```python
from build123d import *

# Parameters (mm, degrees)
SKETCH_1_R              = 5
EXTRUDE_1_DEPTH         = 10
SKETCH_2_R              = 4.501699131
SKETCH_2_R_2            = 2
CUT_EXTRUDE_1_DEPTH     = 0.5
HOLE_WIZARD_M2_21_D     = 2.3
HOLE_WIZARD_M2_21_DEPTH = 2
HOLE_WIZARD_M2_21_TIP   = 0.690989712


with BuildPart() as part:
    # Эскиз1 → Бобышка-Вытянуть1 (new body)
    with BuildSketch(Plane(origin=(0, 0, 0), x_dir=(1, 0, 0), z_dir=(0, 1, 0))):
        Circle(SKETCH_1_R)
    extrude(amount=EXTRUDE_1_DEPTH)

    # Эскиз2 → Вырез-Вытянуть1 (cut)
    with BuildSketch(Plane.XZ):
        Circle(SKETCH_2_R)
        Circle(SKETCH_2_R_2, mode=Mode.SUBTRACT)
    extrude(amount=-CUT_EXTRUDE_1_DEPTH, mode=Mode.SUBTRACT)

    # Сверло под метчик  спиральное M2.21
    with Locations(Plane(origin=(0, 10, 0), x_dir=(1, 0, 0), z_dir=(0, 1, 0))):
        with Locations((0, 0)):
            Hole(HOLE_WIZARD_M2_21_D / 2, depth=HOLE_WIZARD_M2_21_DEPTH)
            with Locations((0, 0, -(HOLE_WIZARD_M2_21_DEPTH + HOLE_WIZARD_M2_21_TIP / 2))):  # 118° drill point
                Cone(0, HOLE_WIZARD_M2_21_D / 2, HOLE_WIZARD_M2_21_TIP, mode=Mode.SUBTRACT)


solid = part.part
```
Source: CAD feature listing. Evaluate the final solid. Frame: model axes, mm. A direction names the side the tool comes from. Round coordinates to 2 decimals unless told otherwise and drop trailing zeros. Write each loop counter-clockwise with the first axis right and the second up, starting at its lowest first coordinate (ties: lowest second). Pieces come first, ordered by that corner, then holes. Notation, with made-up numbers: M -15.75,63.5 L 16.25,63.5 A12 cw 16.25,86.5 Z; hole C 13,72.5 d8. An arc over 180 degrees is marked long. Answer as a JSON object with one key per item and string values. Group by question number.
(1) Reachability of faces 1 (the flat face through (2, 0.5, -1)), 2 (the flat face through (1, 10, 1)), 3 (the cylindrical face through (0.91, 8.99, 0.7)) from +Z, -Z, +X, -X, +Y, -Y: full face, straight path, thin tool, end or side. Return the list, or none.
(2) Section query B-B on z = 3.5. Output: boundary loops of the cut face in (x, y), then the cut area to 3 significant figures.
(3) Mould query, pull axis X, two halves, no side actions, for faces 4 (the flat face through (0, 0, 0)), 5 (the cylindrical face through (-1.08, 4.93, 4.88)), 6 (the cylindrical face through (-0.586, 0.246, 4.463)). Classes: +X half, -X half, draft (parallel to the pull), parting line (faces both ways), or undercut.
(4) First-contact query: pin 1 (2.5 mm diameter, centred on x = 1, z = 0.5, fed in from -Y); pin 2 (1.5 mm diameter, centred on y = 8, z = -1, fed in from +X); pin 3 (1.4 mm diameter, centred on x = 0, z = 0, fed in from +Y); pin 4 (2 mm diameter, centred on x = -1.5, y = 6, fed in from +Z). Flat tips, straight axial feed; report the tip coordinate or a pass-through.
(5) Ray query, line 1 (Z direction, x = 0, y = 0.25); line 2 (Z direction, x = 0, y = 8.65); line 3 (Z direction, x = 0.5, y = 9.25). Return the intervals inside material, ascending. Write a range as [from, to].
(6) Section query A-A on x = -3. Output: boundary loops of the cut face in (y, z).
(7) Section query D-D on x = -1.5. Output: boundary loops of the cut face in (y, z).
(8) Section query C-C on y = 4. Output: boundary loops of the cut face in (x, z).
Computed values:
{
 "1": {"face 1": "-Y", "face 2": "+Z, -Z, +X, -X, +Y", "face 3": "+Y"},
 "2": {"outline": "M -3.57,0 L -2.83,0 L -2.83,0.5 L 2.83,0.5 L 2.83,0 L 3.57,0 L 3.57,10 L -3.57,10 Z", "area": "68.6 mm^2"},
 "3": {"face 4": "draft", "face 5": "parting line", "face 6": "undercut"},
 "4": {"pin 1": "y = 0", "pin 2": "x = 4.99", "pin 3": "y = 7.73", "pin 4": "z = 4.97"},
 "5": {"line 1": "[-5, -4.5], [-2, 2], [4.5, 5]", "line 2": "[-5, -1.15], [1.15, 5]", "line 3": "[-4.97, -1.04], [1.04, 4.97]"},
 "6": {"outline": "M 0,-4 L 10,-4 L 10,4 L 0,4 L 0,3.36 L 0.5,3.36 L 0.5,-3.36 L 0,-3.36 Z"},
 "7": {"outline": "M 0,-4.77 L 10,-4.77 L 10,4.77 L 0,4.77 L 0,4.24 L 0.5,4.24 L 0.5,1.32 L 0,1.32 L 0,-1.32 L 0.5,-1.32 L 0.5,-4.24 L 0,-4.24 Z"},
 "8": {"outline": "C 0,0 d10"}
}
